Input: part model. Units: mm. Frame: model coordinates. Face numbers are marked on the shaded views. A direction names the side the tool comes from. Round coordinates to 2 decimals unless told otherwise and drop trailing zeros. Loops run counter-clockwise (first coordinate to the right, second up) from the corner with the lowest first, then second, coordinate; pieces in that order, holes last. Notation, with made-up numbers: (13, 11.25) -> (69, 11.25) arc R4 cw to (69, 18.25) -> close; hole circle Ø11 at (-2.5, 24.25). An arc over 180 degrees is marked (long way). Answer in a Markdown table with one row per item. Add a question column.
Q1. Pin query (flat end, axial travel): pin 1 (12 mm diameter, centred on y = 18, z = -6, fed in from +X); pin 2 (2 mm diameter, centred on y = 20, z = 2.5, fed in from -X); pin 3 (5 mm diameter, centred on x = 2, z = -2, fed in from -Y). Return the tip coordinate at first contact, or that it passes through.
Q2. Section B-B, the plane x = -9.5. Output: boundary loops of the cut face in (y, z), and give its area (3 significant figures).
Q3. Ray query, L1, parallel to Z at x = 0, y = 20; L2, parallel to Z at x = 0, y = 4.85. Return the intervals inside material, ascending. Write a range as from..to.
Q4. Reachability of the marked faces 1 and 2 from +Z, -Z, +X, -X, +Y, -Y: full face, straight path, thin tool, end or side. Return the list, or none.
Q5. Section D-D, the plane y = 11.5. Output: boundary loops of the cut face in (x, z).
Q6. Section C-C, the plane z = -8.5. Output: boundary loops of the cut face in (x, y).
Q7. Section A-A, the plane y = 3.25. Output: boundary loops of the cut face in (x, z), and give its area (3 significant figures).
```python
from build123d import *

# Parameters (mm, degrees)
CROQUIS1_W              = 36.7
CROQUIS1_H              = 40
CROQUIS1_R              = 4
SALIENTE_EXTRUIR1_DEPTH = 7
CHAFL_N1_SIZE           = 1
CROQUIS3_R              = 6.55
CORTAR_EXTRUIR1_DEPTH   = 2


with BuildPart() as part:
    # Croquis1 → Saliente-Extruir1 (new body)
    with BuildSketch(Plane(origin=(0, 0, 0), x_dir=(1, 0, 0), z_dir=(0, 1, 0))):
        Rectangle(CROQUIS1_W, CROQUIS1_H)
        with Locations(Location((0, 0, 0), (0, 0, 270))):
            Circle(CROQUIS1_R, mode=Mode.SUBTRACT)
    extrude(amount=SALIENTE_EXTRUIR1_DEPTH)

    # Croquis2 → Revolución1 (revolve)
    with BuildSketch(Plane(origin=(0, 0, 0), x_dir=(0, 0, -1), z_dir=(1, 0, 0))):
        Polygon((7, 7), (7, 12), (5.5, 12), (5.5, 15), (7, 15), (7, 18), (5.5, 18), (5.5, 21), (7, 22.5), (7, 24.5), (4, 24.5), (4, 7), align=None)
    revolve(axis=Axis((0, 7, 0), (0, 1, 0)))

    # Chaflán1
    chafl_n1_edges = [part.edges().sort_by_distance(p)[0] for p in [
        (0, 12, 7),
        (0, 15, 7),
    ]]
    chamfer(chafl_n1_edges, length=CHAFL_N1_SIZE)

    # Croquis3 → Cortar-Extruir1 (cut)
    with BuildSketch(Plane.XZ):
        with Locations(Location((0, 0, 0), (0, 0, 270))):
            Circle(CROQUIS3_R)
    extrude(amount=-CORTAR_EXTRUIR1_DEPTH, mode=Mode.SUBTRACT)


solid = part.part
```
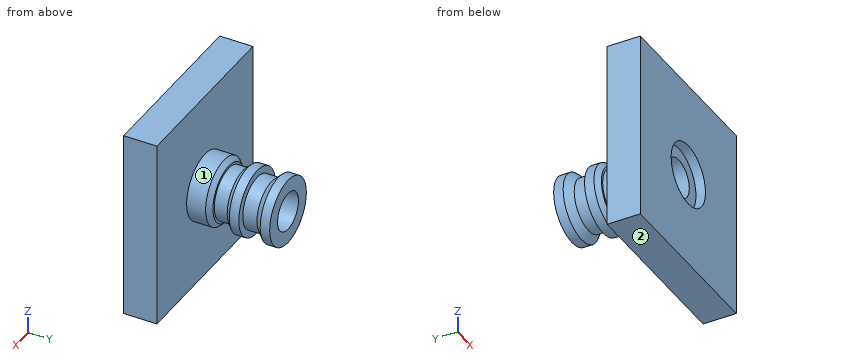
Answer block:
| question | item | result |
|---|---|---|
| 1 | pin 1 | x = 7 |
| 1 | pin 2 | x = -5.29 |
| 1 | pin 3 | y = 2 |
| 2 | outline | (0, -20) -> (7, -20) -> (7, 20) -> (0, 20) -> close |
| 2 | area | 280 mm^2 |
| 3 | L1 | -5.5..-4, 4..5.5 |
| 3 | L2 | -20..-4, 4..20 |
| 4 | face 1 | +Y |
| 4 | face 2 | -Z, +X, -X, +Y, -Y |
| 5 | outline | circle Ø13 at (0, 0); hole circle Ø8 at (0, 0) |
| 6 | outline | (-18.35, 0) -> (18.35, 0) -> (18.35, 7) -> (-18.35, 7) -> close |
| 7 | outline | (-18.35, -20) -> (18.35, -20) -> (18.35, 20) -> (-18.35, 20) -> close; hole circle Ø8 at (0, 0) |
| 7 | area | 1,420 mm^2 |
